The listing builds one solid part. Answer for the finished solid, in the listing's coordinates (mm). A direction names the side the tool comes from. Round coordinates to 2 decimals unless told otherwise and drop trailing zeros. Order: outer loops, then holes, each group sorted by start corner. A loop starts at its lowest first (then second) coordinate and runs counter-clockwise, first axis right, second up. Notation, with made-up numbers: (-6.5, 77) -> (29.5, 77) arc R20 ccw to (29.5, 111) -> close; hole circle Ø5 at (67, 75.25). An arc over 180 degrees is marked (long way). Return JSON: item names as keys, results as strings. Group by question number.
(1) Consider line 1 (X direction, y = 5.75, z = -23.5); line 2 (Z direction, x = -23.5, y = 8.75); line 3 (X direction, y = 16, z = -15). Determine where each line is inside the solid, lowest interval first. Write a range as [from, to].
(2) Determine the mould class of faces 1 (the face through (-29, 5, -19)), 2 (the face through (30, 9, 0)), 3 (the face through (-24, 2, 24)) for opening direction Y: +Y half, -Y half, draft (parallel to the pull), parting line (faces both ways), or undercut.
(3) The part is cut by section A-A (y = 13). Determine the outline of the cut face in (x, z).
(4) Each of these flat-tipped pins is pushed along its axis until it touches: pin 1 (4 mm diameter, centred on x = -16, z = 20.5, fed in from -Y); pin 2 (0.6 mm diameter, centred on x = -28, z = 28.5, fed in from +Y); pin 3 (1.1 mm diameter, centred on x = -23, z = -23.5, fed in from +Y); pin 4 (5 mm diameter, centred on x = -18, z = -18, fed in from +Y). Where does it stop, or does it pass through?
(5) Which of the six approach directions +Z, -Z, +X, -X, +Y, -Y give full straight-line access (tool end or side, diameter ignored) to faces 4 (the face through (0, 9, -30)), 5 (the face through (-28, 15, -29))?
(6) The part is cut by section B-B (z = -17). Determine the outline of the cut face in (x, y).
(7) The part is cut by section C-C (y = 8). Count the separate pieces of the cut face and the enclosed holes in it, plus the area to 3 significant figures.
(8) The part is cut by section D-D (x = 19.5). Determine the outline of the cut face in (y, z), plus the area to 3 significant figures.
from build123d import *

# Parameters (mm, degrees)
SKETCH_1_W          = 56
SKETCH_1_H          = 56
EXTRUDE_1_DEPTH     = 2
SKETCH_2_R          = 1.8
EXTRUDE_2_DEPTH     = 8.6
SKETCH_3_R          = 1
CUT_EXTRUDE_1_DEPTH = 8.6
SKETCH_5_W          = 58
SKETCH_5_H          = 2
EXTRUDE_3_DEPTH     = 19
SKETCH_6_W          = 2
SKETCH_6_H          = 58
EXTRUDE_4_DEPTH     = 19
SKETCH_7_W          = 58
SKETCH_7_H          = 2
EXTRUDE_5_DEPTH     = 19
SKETCH_8_W          = 2
SKETCH_8_H          = 58
EXTRUDE_6_DEPTH     = 19
SKETCH_9_R          = 2
CUT_EXTRUDE_2_DEPTH = 2
SKETCH_10_R         = 1.6
EXTRUDE_7_DEPTH     = 17
SKETCH_11_R         = 1
CUT_EXTRUDE_3_DEPTH = 9
FILLET_1_R          = 1


with BuildPart() as part:
    # Sketch 1 → Extrude 1 (new body)
    with BuildSketch(Plane(origin=(0, 0, 0), x_dir=(1, 0, 0), z_dir=(0, 1, 0))):
        Rectangle(SKETCH_1_W, SKETCH_1_H)
    extrude(amount=EXTRUDE_1_DEPTH)

    # Sketch 2 → Extrude 2 (add)
    with BuildSketch(Plane(origin=(0, 2, 0), x_dir=(1, 0, 0), z_dir=(0, 1, 0))):
        with Locations((-23.5, -23.5)):
            Circle(SKETCH_2_R)
        with Locations((-23.5, 23.5)):
            Circle(SKETCH_2_R)
        with Locations((23.5, 23.5)):
            Circle(SKETCH_2_R)
        with Locations((23.5, -23.5)):
            Circle(SKETCH_2_R)
    extrude(amount=EXTRUDE_2_DEPTH)

    # Sketch 3 → Cut-Extrude 1 (cut)
    with BuildSketch(Plane(origin=(0, 10.6, 0), x_dir=(1, 0, 0), z_dir=(0, 1, 0))):
        with Locations((-23.5, 23.5)):
            Circle(SKETCH_3_R)
        with Locations((23.5, 23.4724717)):
            Circle(SKETCH_3_R)
        with Locations((23.5, -23.5)):
            Circle(SKETCH_3_R)
        with Locations((-23.5, -23.516051304)):
            Circle(SKETCH_3_R)
    extrude(amount=-CUT_EXTRUDE_1_DEPTH, mode=Mode.SUBTRACT)



with BuildPart() as body_2:
    # Sketch 5 → Extrude 3 (new body)
    with BuildSketch(Plane.XZ):
        with Locations((1, -29)):
            Rectangle(SKETCH_5_W, SKETCH_5_H)
    extrude(amount=-EXTRUDE_3_DEPTH)


with BuildPart() as part_1:
    add(part.part)

    add(body_2.part)  # Extrude 4 merges body 2
    # Sketch 6 → Extrude 4 (add)
    with BuildSketch(Plane.XZ):
        with Locations((29, 1)):
            Rectangle(SKETCH_6_W, SKETCH_6_H)
    extrude(amount=-EXTRUDE_4_DEPTH)



with BuildPart() as body_2_2:
    # Sketch 7 → Extrude 5 (new body)
    with BuildSketch(Plane.XZ):
        with Locations((-1, 29)):
            Rectangle(SKETCH_7_W, SKETCH_7_H)
    extrude(amount=-EXTRUDE_5_DEPTH)


with BuildPart() as part_2:
    add(part_1.part)

    add(body_2_2.part)  # Extrude 6 merges body 2 2
    # Sketch 8 → Extrude 6 (add)
    with BuildSketch(Plane.XZ):
        with Locations((-29, -1)):
            Rectangle(SKETCH_8_W, SKETCH_8_H)
    extrude(amount=-EXTRUDE_6_DEPTH)

    # Sketch 9 → Cut-Extrude 2 (cut)
    with BuildSketch(Plane.ZY.offset(30)):
        with Locations((-17, 5)):
            Circle(SKETCH_9_R)
    extrude(amount=-CUT_EXTRUDE_2_DEPTH, mode=Mode.SUBTRACT)

    # Sketch 10 → Extrude 7 (add)
    with BuildSketch(Plane(origin=(0, 2, 0), x_dir=(1, 0, 0), z_dir=(0, 1, 0))):
        with Locations((-28, 28)):
            Circle(SKETCH_10_R)
        with Locations((28, 28)):
            Circle(SKETCH_10_R)
        with Locations((28, -28)):
            Circle(SKETCH_10_R)
        with Locations((-28, -28)):
            Circle(SKETCH_10_R)
    extrude(amount=EXTRUDE_7_DEPTH)

    # Sketch 11 → Cut-Extrude 3 (cut)
    with BuildSketch(Plane(origin=(0, 19, 0), x_dir=(1, 0, 0), z_dir=(0, 1, 0))):
        with Locations((-28, 28)):
            Circle(SKETCH_11_R)
        with Locations((28, 28)):
            Circle(SKETCH_11_R)
        with Locations((-28, -28)):
            Circle(SKETCH_11_R)
        with Locations((28, -28)):
            Circle(SKETCH_11_R)
    extrude(amount=-CUT_EXTRUDE_3_DEPTH, mode=Mode.SUBTRACT)

    # Fillet 1
    fillet_1_edges = [part_2.edges().sort_by_distance(p)[0] for p in [
        (-30, 9.5, 30),
        (30, 9.5, 30),
        (30, 9.5, -30),
        (-30, 9.5, -30),
    ]]
    fillet(fillet_1_edges, radius=FILLET_1_R)


solid = part_2.part
Answer below:
{
 "1": {"line 1": "x = [-30, -28], [-25.3, -24.5], [-22.5, -21.7], [21.7, 22.5], [24.5, 25.3], [28, 30]", "line 2": "z = [-30, -28], [-25.3, -24.5], [-22.5, -21.7], [21.7, 22.52], [24.52, 25.3], [28, 30]", "line 3": "x = [-30, -28], [28, 30]"},
 "2": {"face 1": "undercut", "face 2": "draft", "face 3": "+Y half"},
 "3": {"outline": "(-30, -29) arc R1 ccw to (-29, -30) -> (29, -30) arc R1 ccw to (30, -29) -> (30, 29) arc R1 ccw to (29, 30) -> (-29, 30) arc R1 ccw to (-30, 29) -> close; hole circle Ø2 at (-28, -28); hole circle Ø2 at (-28, 28); hole (-28, -26.4) arc R1.6 cw to (-26.4, -28) -> (26.4, -28) arc R1.6 cw to (28, -26.4) -> (28, 26.4) arc R1.6 cw to (26.4, 28) -> (-26.4, 28) arc R1.6 cw to (-28, 26.4) -> close; hole circle Ø2 at (28, -28); hole circle Ø2 at (28, 28)"},
 "4": {"pin 1": "stops at y = 0", "pin 2": "stops at y = 10", "pin 3": "stops at y = 10.6", "pin 4": "stops at y = 2"},
 "5": {"face 4": "-Z, +X, -X, +Y, -Y", "face 5": "+Y"},
 "6": {"outline": "(-30, 0) -> (30, 0) -> (30, 19) -> (28, 19) -> (28, 2) -> (-28, 2) -> (-28, 3) -> (-30, 3) -> close; (-30, 7) -> (-28, 7) -> (-28, 19) -> (-30, 19) -> close"},
 "7": {"separate pieces": "5", "enclosed holes": "5", "area": "499 mm²"},
 "8": {"outline": "(0, -30) -> (19, -30) -> (19, -28) -> (2, -28) -> (2, 28) -> (19, 28) -> (19, 30) -> (0, 30) -> close", "area": "188 mm²"}
}
